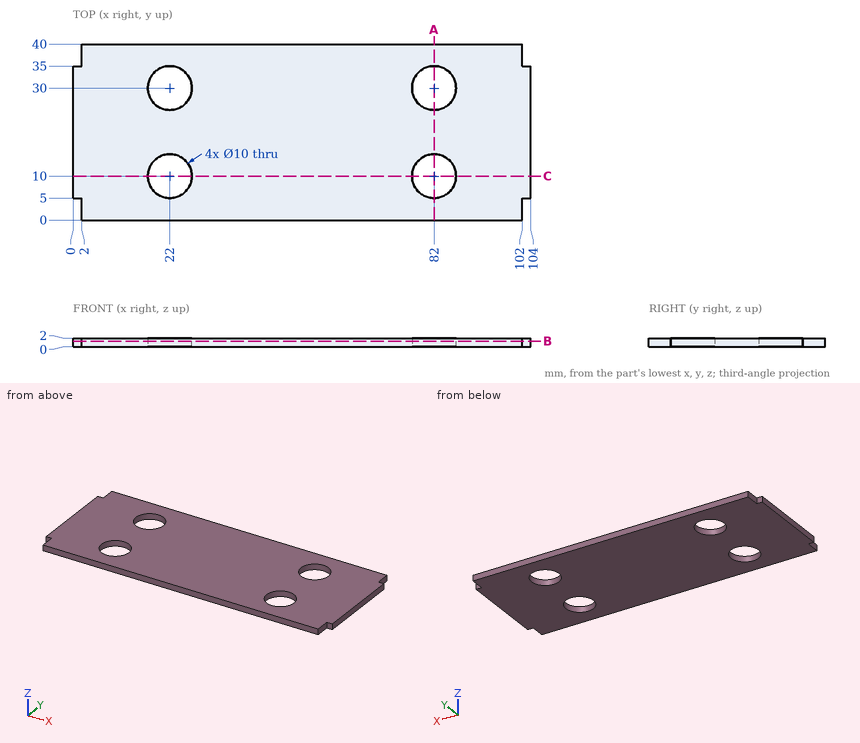
Source: three-view drawing plus pictorial views. Frame: mm from the lowest corner of the part. Give positions to 0.01 mm unless a question says otherwise; leave off trailing zeros. Loops run counter-clockwise (first coordinate to the right, second up) from the corner with the lowest first, then second, coordinate; pieces in that order, holes last.
1) Section query A-A on x = 82. Return the cut outline in (y, z).
A:
outline: (0, 0) - (5, 0) - (5, 2) - (0, 2) - close; (15, 0) - (25, 0) - (25, 2) - (15, 2) - close; (35, 0) - (40, 0) - (40, 2) - (35, 2) - close
2) Line query: L1, parallel to Y at x = 82, z = 1.5; L2, parallel to X at y = 30, z = 1.15; L3, parallel to X at y = 34, z = 0.9. Output: solid intervals per line, ascending.
A:
L1: y = 0 to 5, 15 to 25, 35 to 40
L2: x = 0 to 17, 27 to 77, 87 to 104
L3: x = 0 to 19, 25 to 79, 85 to 104
3) Section query B-B on z = 1.3. Return the cut outline in (x, y), and give its area (3 significant figures).
A:
outline: (0, 5) - (2, 5) - (2, 0) - (102, 0) - (102, 5) - (104, 5) - (104, 35) - (102, 35) - (102, 40) - (2, 40) - (2, 35) - (0, 35) - close; hole circle Ø10 at (22, 10); hole circle Ø10 at (22, 30); hole circle Ø10 at (82, 10); hole circle Ø10 at (82, 30)
area: 3,810 mm2
4) Section query C-C on y = 10. Return the cut outline in (x, z), and give its area (3 significant figures).
A:
outline: (0, 0) - (17, 0) - (17, 2) - (0, 2) - close; (27, 0) - (77, 0) - (77, 2) - (27, 2) - close; (87, 0) - (104, 0) - (104, 2) - (87, 2) - close
area: 168 mm2
5) Contact query for flat-ended pins moving along their axis: pin 1 (0.6 mm diameter, centred on x = 103, z = 1, fed in from +Y); pin 2 (1 mm diameter, centred on x = 103.5, z = 1.5, fed in from -Y); pin 3 (0.6 mm diameter, centred on y = 37, z = 0.5, fed in from -X). Output: stop coordinate, or through.
A:
pin 1: stops at y = 35
pin 2: stops at y = 5
pin 3: stops at x = 2
